Autodesk Inventor part; units mm, degrees
ref_plane "YZ Plane" through (0, 0, 0) normal (1, 0, 0) x (0, 1, 0)
ref_plane "XZ Plane" through (0, 0, 0) normal (0, 1, 0) x (-1, 0, 0)
ref_plane "XY Plane" through (0, 0, 0) normal (0, 0, 1) x (1, 0, 0)
sketch "Sketch3" plane through (0, 0, 0) normal (0, 0, 1) x (1, 0, 0)
  line L0 (0, 0) -> (0, 42)
  line L1 (11.25, 0) -> (11.25, 12)
  line L2 (11.25, 12) -> (19, 12)
  line L3 (19, 12) -> (25.6098, 42)
  line L4 (25.6098, 42) -> (31.7537, 42)
  line L5 (31.7537, 42) -> (22.5, 0)
  line L6 (22.5, 0) -> (11.25, 0)
  dimension "d3" = 6
  dimension "d4" = 42
  dimension "d5" = 12
  dimension "d6" = 22.5
  dimension "d7" = 45
  dimension "d8" = 38
  dimension "d9" = 63.5073
revolve "Revolution1" add sketch "Sketch3" angle 360 about axis through (0, 0, 0) along (0, 1, 0)
sketch "Sketch4" plane through (0, 0, 0) normal (0, 0, 1) x (1, 0, 0)
  line L0 (31.7537, 42) -> (-31.7537, 42)
  circle A0 centre (0, 42) radius 5
  point P0 (0, 0)
  dimension "d11" = 10
extrude "Extrusion2" cut sketch "Sketch4" along normal through all
pattern_circular "Circular Pattern1" count 4 over 360 about axis through (0, -10, 0) along (0, 1, 0) of "Extrusion2"
properties part number "cup" material "Steel, Cast"
For this review, take the finished solid that the model builds, in its own axes (mm). A direction names the side the tool comes from. Coordinates: 2 decimals unless noted, no trailing zeros. Order: outer loops, then holes, each group sorted by start corner. A loop starts at its lowest first (then second) coordinate and runs counter-clockwise, first axis right, second up. Notation, with made-up numbers: (37, -33.75) -> (42, -33.75) arc R11 ccw to (42, -26.75) -> close; hole circle Ø6 at (86.5, 50). An arc over 180 degrees is marked (long way). Use CSV: the item, a comma, the result in double quotes. Start each with the question number.
Item 1: Insertion check: pin 1 (10 mm diameter, centred on x = -16.5, y = 25.5, fed in from -Z); pin 2 (4 mm diameter, centred on y = 13, z = 8.5, fed in from -X); pin 3 (10 mm diameter, centred on y = 26, z = 1, fed in from -X). Each pin has a flat end and moves straight along its axis. Give the tip position at first contact, or say it passes through.
Item 2: For faces 4 (the face through (0, 37, -28)), 5 (the face through (8.2, 12, 8.2)), list the 3-axis set-ups (+Z, -Z, +X, -X, +Y, -Y) from which the entire face can be reached by the end or side of a thin tool; tool diameter is ignored.
Item 3: We need section B-B, the plane x = 0. Give the boundary of the cut face in (y, z), then the cut area to 3 significant figures.
Item 4: We need section A-A, the plane z = 0. Give the boundary of the cut face in (x, y), then the cut area to 3 significant figures.
Item 5: We need section D-D, the plane y = 23.5. Give the boundary of the cut face in (x, z), then the cut area to 3 significant figures.
Item 6: Wall thickness on probe 1 along X at (y, z) = (29.5, 1); probe 2 along X at (y, z) = (23, -11); probe 3 along Z at (x, y) = (3.5, 21): over which ranges is each line inside the solid? List them lowest first.
Item 7: We need section C-C, the plane y = 31. Give the boundary of the cut face in (x, z).
Item 8: Draft analysis for pull direction Z (two halves, no side actions). For faces 1 (the face through (5.19, 6.08, 9.98)), 2 (the face through (19, 42, -18)), 3 (the face through (12.073, 16.627, 23.211)), state which applies: pulls with the +Z half, pulls with the -Z half, needs draft (parallel to the pull), parting line crosses it, or undercut.
Derived:
1,pin 1,"stops at z = -25.96"
1,pin 2,"stops at x = -24.68"
1,pin 3,"stops at x = -29.32"
2,face 4,"+Z, -Z, +Y"
2,face 5,"+Y"
3,outline,"(0, -22.5) -> (37, -30.65) -> (37, -24.51) -> (12, -19) -> (12, -11.25) -> (0, -11.25) -> close; (0, 11.25) -> (12, 11.25) -> (12, 19) -> (37, 24.51) -> (37, 30.65) -> (0, 22.5) -> close"
3,area,"609 mm^2"
4,outline,"(-30.65, 37) -> (-22.5, 0) -> (-11.25, 0) -> (-11.25, 12) -> (-19, 12) -> (-24.51, 37) -> close; (11.25, 0) -> (22.5, 0) -> (30.65, 37) -> (24.51, 37) -> (19, 12) -> (11.25, 12) -> close"
4,area,"609 mm^2"
5,outline,"circle Ø55.36 at (0, 0); hole circle Ø43.07 at (0, 0)"
5,area,"950 mm^2"
6,probe 1,"x = -28.98 to -22.83, 22.83 to 28.98"
6,probe 2,"x = -25.28 to -18.38, 18.38 to 25.28"
6,probe 3,"z = -26.9 to -20.69, 20.69 to 26.9"
7,outline,"circle Ø58.66 at (0, 0); hole circle Ø46.37 at (0, 0)"
8,face 1,"undercut"
8,face 2,"needs draft"
8,face 3,"parting line crosses it"
